Part model, mm, in its own coordinate system. A direction names the side the tool comes from. Round coordinates to 2 decimals unless told otherwise and drop trailing zeros. Order: outer loops, then holes, each group sorted by start corner. A loop starts at its lowest first (then second) coordinate and runs counter-clockwise, first axis right, second up. Notation, with made-up numbers: M 43,74.5 L 75,74.5 A15 cw 75,97.5 Z; hole C 84.25,67.5 d2. An arc over 180 degrees is marked long. Write each question's results on one line, items separated by ' | '. Start each with the question number.
1. Two-plate mould, pull along Y, no slides. Class faces 1 (the face through (5.6, 8.8, 5.6)), 2 (the face through (13.4, 5.07, 2.46)), 3 (the face through (11, 5, 5)): +Y half, -Y half, draft (parallel to the pull), parting line (faces both ways), or undercut.
2. Band-saw the part on D-D, the plane z = 15. List the corners of the cut face in (x, y).
3. Band-saw the part on C-C, the plane x = 15. List the corners of the cut face in (y, z).
4. Drop flat-ended pins along their axis: pin 1 Ø4.5 at (y, z) = (6, 12) entering from +X; pin 2 Ø8 at (x, z) = (11.5, 8) entering from -Y; pin 3 Ø2 at (x, z) = (14, 4) entering from -Y; pin 4 Ø3 at (x, y) = (15, 5) entering from +Z. Give the stop position or say it passes through.
5. Band-saw the part on A-A, the plane y = 5. List the corners of the cut face in (x, z).
6. Which spindle directions (+Z, -Z, +X, -X, +Y, -Y) get a long thin tool onto all of the face, cutting with end or side? Do faces 4 (the face through (4, 2, 12)), 5 (the face through (19, 8, 1)), 6 (the face through (12, 8, 4)). Say none if no direction does.
7. Probe L1, parallel to Z at x = 1.4, y = 5; L2, parallel to Z at x = 13.25, y = 3.25; L3, parallel to X at y = 2.75, z = 2.25. List the from-to ranges inside material, lowest first. Write a range as [from, to].
8. Band-saw the part on B-B, the plane z = 1.75. List the corners of the cut face in (x, y).
```python
from build123d import *

# Parameters (mm, degrees)
SKIZZE1_W                       = 15
SKIZZE1_H                       = 10
SKIZZE1_R                       = 1.6
AUFSATZ_LINEAR_AUSTRAGEN1_DEPTH = 5
SKIZZE1_9_W                     = 5
SKIZZE1_9_H                     = 10
AUFSATZ_LINEAR_AUSTRAGEN2_DEPTH = 20
SKIZZE3_R                       = 1.6
SCHNITT_LINEAR_AUSTRAGEN2_DEPTH = 20
FASE1_SIZE                      = 3


with BuildPart() as part:
    # Skizze1 → Aufsatz-Linear austragen1 (new body)
    with BuildSketch(Plane.XY):
        with Locations((12.5, 5)):
            Rectangle(SKIZZE1_W, SKIZZE1_H)
        with Locations((15, 5)):
            Circle(SKIZZE1_R, mode=Mode.SUBTRACT)
    extrude(amount=AUFSATZ_LINEAR_AUSTRAGEN1_DEPTH)

    # Skizze1_9 → Aufsatz-Linear austragen2 (add)
    with BuildSketch(Plane.XY):
        with Locations((2.5, 5)):
            Rectangle(SKIZZE1_9_W, SKIZZE1_9_H)
    extrude(amount=AUFSATZ_LINEAR_AUSTRAGEN2_DEPTH)

    # Skizze3 → Schnitt-Linear austragen2 (cut)
    with BuildSketch(Plane(origin=(5, 0, 0), x_dir=(0, 0, -1), z_dir=(1, 0, 0))):
        with Locations(Location((-15, 5, 0), (0, 0, 90))):
            Circle(SKIZZE3_R)
    extrude(amount=-SCHNITT_LINEAR_AUSTRAGEN2_DEPTH, mode=Mode.SUBTRACT)

    # Fase1
    fase1_edges = [part.edges().sort_by_distance(p)[0] for p in [
        (12.5, 0, 5),
        (20, 10, 2.5),
        (20, 0, 2.5),
        (20, 5, 5),
        (5, 5, 20),
        (5, 0, 12.5),
        (2.5, 10, 20),
        (5, 10, 12.5),
        (12.5, 10, 5),
        (2.5, 0, 20),
        (5, 5, 5),
    ]]
    chamfer(fase1_edges, length=FASE1_SIZE)


solid = part.part
```
Solution:
1) face 1: +Y half | face 2: undercut | face 3: draft
2) outline: M 0,0 L 2,0 L 5,3 L 5,3.4 L 0,3.4 Z; M 0,6.6 L 5,6.6 L 5,7 L 2,10 L 0,10 Z
3) outline: M 0,0 L 3.4,0 L 3.4,5 L 3,5 L 0,2 Z; M 6.6,0 L 10,0 L 10,2 L 7,5 L 6.6,5 Z
4) pin 1: x = 5 | pin 2: y = 2 | pin 3: y = 1 | pin 4: through
5) outline: M 0,0 L 13.4,0 L 13.4,5 L 8,5 L 5,8 L 5,13.4 L 0,13.4 Z; M 0,16.6 L 5,16.6 L 5,17 L 2,20 L 0,20 Z; M 16.6,0 L 20,0 L 20,2 L 17,5 L 16.6,5 Z
6) face 4: +Z, +X, -Y | face 5: +Z, -Z, +X, +Y | face 6: +Z, +X, +Y
7) L1: [0, 13.4], [16.6, 20] | L2: [0, 5] | L3: [0, 19.5]
8) outline: M 0,0 L 17,0 L 20,3 L 20,7 L 17,10 L 0,10 Z; hole C 15,5 d3.2
